from build123d import *

# Parameters (mm, degrees)
F4_D     = 5
F4_DEPTH = 11.06
F4_TIP   = 1.5021515476
F7_D     = 5
F7_DEPTH = 11.06
F7_TIP   = 1.5021515476


with BuildPart() as f1:
    # F0 (on Front) → F1 (revolve)
    with BuildSketch(Plane.XZ):
        Polygon((0, 25.4), (0, 11.0109), (18.1102, 11.0109), (18.1102, 17.5514), (8.1026, 17.5514), (8.1026, 25.4), align=None)
    revolve(axis=Axis((12.2365328816, 0, 0), (1, 0, 0)))

    # F4
    with Locations(Plane.XZ.offset(17.5514)):
        with Locations((13.1064, 0)):
            Hole(F4_D / 2, depth=F4_DEPTH)
            with Locations((0, 0, -(F4_DEPTH + F4_TIP / 2))):  # 118° drill point
                Cone(0, F4_D / 2, F4_TIP, mode=Mode.SUBTRACT)

    # F7
    with Locations(Plane.XY.offset(17.5514)):
        with Locations((13.1064, 0)):
            Hole(F7_D / 2, depth=F7_DEPTH)
            with Locations((0, 0, -(F7_DEPTH + F7_TIP / 2))):  # 118° drill point
                Cone(0, F7_D / 2, F7_TIP, mode=Mode.SUBTRACT)


solid = f1.part
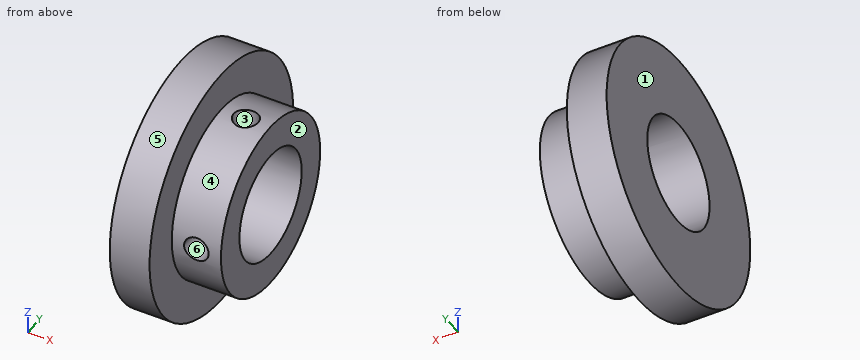
Geometry check sheet. Reference: the model listing, model coordinates, mm. Face numbers are marked on the shaded views. A direction names the side the tool comes from. Give positions to 0.01 mm unless a question says otherwise; leave off trailing zeros. Loops run counter-clockwise (first coordinate to the right, second up) from the corner with the lowest first, then second, coordinate; pieces in that order, holes last. Notation, with made-up numbers: (87.25, 57.5) -> (135.25, 57.5) arc R25 cw to (135.25, 81.5) -> close; hole circle Ø9 at (2.5, -5). An arc over 180 degrees is marked (long way). Answer in a Markdown table with one row per item. Add a question column.
1) Gauge pin test, flat ends, axial feed: P1, Ø3, axis at x = 6.5, z = 16, coming from the +Y side; P2, Ø10, axis at x = 3.5, y = -7, coming from the +Z side; P3, Ø6, axis at x = 2, y = -20, coming from the -Z side. Record the tip position at first contact, or that the pin passes through.
2) Cross-section at A-A on y = 0. Record the boundary of the cut face in (x, z), and give its area (3 significant figures).
3) Set-up check for the marked faces 4, 5 and 6: record each of +Z, -Z, +X, -X, +Y, -Y from which the full face is reachable in a straight line by a thin tool's end or side.
4) Cross-section at D-D on y = 9.5. Record the boundary of the cut face in (x, z).
5) Cross-section at B-B on z = 0. Record the boundary of the cut face in (x, y).
6) Material ranges on probe 1 along X at (y, z) = (-11.75, 0); probe 2 along Y at (x, z) = (7.5, 0); probe 3 along Z at (x, y) = (6, -2), recorded low to high. Write a range as from..to.
7) Draft check along X on the marked faces 1, 2 and 3. Enter one of: pulls with the +X half, pulls with the -X half, needs draft (parallel to the pull), parting line crosses it, or undercut.
8) Cross-section at C-C on x = 13.25. Record the boundary of the cut face in (y, z).
Outcome:
| question | item | result |
|---|---|---|
| 1 | P1 | stops at y = 20.85 |
| 1 | P2 | stops at z = 25.32 |
| 1 | P3 | stops at z = -18.87 |
| 2 | outline | (0, -25.4) -> (8.1, -25.4) -> (8.1, -17.55) -> (18.11, -17.55) -> (18.11, -11.01) -> (0, -11.01) -> close; (0, 11.01) -> (10.61, 11.01) -> (10.61, 17.55) -> (8.1, 17.55) -> (8.1, 25.4) -> (0, 25.4) -> close; (15.61, 11.01) -> (18.11, 11.01) -> (18.11, 17.55) -> (15.61, 17.55) -> close |
| 2 | area | 331 mm^2 |
| 3 | face 4 | +X |
| 3 | face 5 | +X, -X |
| 3 | face 6 | -Y |
| 4 | outline | (0, -23.56) -> (8.1, -23.56) -> (8.1, -14.76) -> (18.11, -14.76) -> (18.11, -5.57) -> (0, -5.57) -> close; (0, 5.57) -> (18.11, 5.57) -> (18.11, 14.76) -> (8.1, 14.76) -> (8.1, 23.56) -> (0, 23.56) -> close |
| 5 | outline | (0, -25.4) -> (8.1, -25.4) -> (8.1, -17.55) -> (10.61, -17.55) -> (10.61, -11.01) -> (0, -11.01) -> close; (0, 11.01) -> (18.11, 11.01) -> (18.11, 17.55) -> (8.1, 17.55) -> (8.1, 25.4) -> (0, 25.4) -> close; (15.61, -17.55) -> (18.11, -17.55) -> (18.11, -11.01) -> (15.61, -11.01) -> close |
| 6 | probe 1 | x = 0..10.61, 15.61..18.11 |
| 6 | probe 2 | y = -25.4..-11.01, 11.01..25.4 |
| 6 | probe 3 | z = -25.32..-10.83, 10.83..25.32 |
| 7 | face 1 | pulls with the -X half |
| 7 | face 2 | pulls with the +X half |
| 7 | face 3 | undercut |
| 8 | outline | (-17.37, -2.5) arc R17.55 ccw (long way) to (2.5, 17.37) -> (2.5, 10.72) arc R11.01 cw (long way) to (-10.72, -2.5) -> close; (-17.37, 2.5) -> (-10.72, 2.5) arc R11.01 cw to (-2.5, 10.72) -> (-2.5, 17.37) arc R17.55 ccw to start |
